The model under review builds one solid part; all positions refer to its coordinate system, in mm. A direction names the side the tool comes from. Coordinates: 2 decimals unless noted, no trailing zeros. Loops run counter-clockwise (first coordinate to the right, second up) from the corner with the lowest first, then second, coordinate; pieces in that order, holes last. Notation, with made-up numbers: (53, 71.5) - (92, 71.5) arc R15 cw to (92, 80.5) - close; hole circle Ø7 at (-7, 60.25). An arc over 180 degrees is marked (long way). One line per item, written item: value. Start each with the question number.
1. To check wall thickness, follow line 1 (X direction, y = 1.85, z = -15); line 2 (X direction, y = 2.3, z = -28); line 3 (Z direction, x = 22, y = 2.5). State the ranges of each line that lie inside material, in increasing order.
2. For faces 1 (the face through (10, 2, -2)), 2 (the face through (7.73, 2.03, -33.99)), 3 (the face through (4, 2, -23)), list the 3-axis set-ups (+Z, -Z, +X, -X, +Y, -Y) from which the entire face can be reached by the end or side of a thin tool; tool diameter is ignored.
3. Insertion check: P1, Ø2, axis at x = 22, y = 2.5, coming from the +Z side; P2, Ø1.2, axis at y = 2, z = -2, coming from the -X side; P3, Ø1.2, axis at y = 3, z = -6.5, coming from the +X side. Each pin has a flat end and moves straight along its axis. Give the tip position at first contact, or say it passes through.
4. We need section A-A, the plane z = -2. Give the boundary of the cut face in (x, y), then the cut area to 3 significant figures.
5. We need section B-B, the plane x = 15. Give the boundary of the cut face in (y, z).
6. Mouldability with a two-part tool opening along Z and no side actions: class faces 4 (the face through (29.14, 2.03, -42.1)), 5 (the face through (15, 2, 0)), 6 (the face through (15.07, 2.03, -29.5)), 7 (the face through (20, 2, -2)) as +Z half, -Z half, draft (parallel to the pull), parting line (faces both ways), or undercut.
7. We need section C-C, the plane x = 21.25. Give the boundary of the cut face in (y, z).
8. We need section D-D, the plane y = 1.8. Count the separate pieces of the cut face and the enclosed holes in it, then the cut area to 3 significant figures.
from build123d import *

# Parameters (mm, degrees)
SKETCH1_W           = 10
SKETCH1_H           = 4
SKETCH1_W_2         = 4
SKETCH1_H_2         = 10
BOSS_EXTRUDE1_DEPTH = 4
SKETCH3_W           = 30
SKETCH3_H           = 4
BOSS_EXTRUDE2_DEPTH = 13
SKETCH4_R           = 2.2
CUT_EXTRUDE2_DEPTH  = 10
FILLET1_R           = 3
FILLET2_R           = 4
SKETCH6_R           = 1.5
CUT_EXTRUDE3_DEPTH  = 10


with BuildPart() as part:
    # Sketch1 → Boss-Extrude1 (new body)
    with BuildSketch(Plane(origin=(0, 0, 0), x_dir=(1, 0, 0), z_dir=(0, 1, 0))):
        Polygon((4, 10), (4, 4), (10, 4), (20, 4), (26, 4), (26, 10), (26, 20), (26, 26), (20, 26), (10, 26), (4, 26), (4, 20), align=None)
        with Locations((15, 2)):
            Rectangle(SKETCH1_W, SKETCH1_H)
        with Locations((28, 15)):
            Rectangle(SKETCH1_W_2, SKETCH1_H_2)
        with Locations((15, 28)):
            Rectangle(SKETCH1_W, SKETCH1_H)
        with Locations((2, 15)):
            Rectangle(SKETCH1_W_2, SKETCH1_H_2)
    extrude(amount=BOSS_EXTRUDE1_DEPTH)

    # Sketch3 → Boss-Extrude2 (add)
    with BuildSketch(Plane(origin=(0, 0, -30), x_dir=(-1, 0, 0), z_dir=(0, 0, -1))):
        with Locations((-15, 2)):
            Rectangle(SKETCH3_W, SKETCH3_H)
    extrude(amount=BOSS_EXTRUDE2_DEPTH)

    # Sketch4 → Cut-Extrude2 (cut)
    with BuildSketch(Plane(origin=(0, 4, 0), x_dir=(1, 0, 0), z_dir=(0, 1, 0))):
        with Locations((24, 36.5)):
            Circle(SKETCH4_R)
        with Locations((6, 36.5)):
            Circle(SKETCH4_R)
        Polygon((9.146625176, 38.868807717), (3.631192283, 33.353374824), (2.853374824, 34.131192283), (8.368807717, 39.646625176), align=None)
        Polygon((21.684225292, 39.699658185), (27.199658185, 34.184225292), (26.315774708, 33.300341815), (20.800341815, 38.815774708), align=None)
        Polygon((8.368807717, 33.353374824), (9.146625176, 34.131192283), (3.631192283, 39.646625176), (2.853374824, 38.868807717), align=None)
        Polygon((20.800341815, 34.184225292), (21.684225292, 33.300341815), (27.199658185, 38.815774708), (26.315774708, 39.699658185), align=None)
    extrude(amount=-CUT_EXTRUDE2_DEPTH, mode=Mode.SUBTRACT)

    # Fillet1
    fillet1_edges = [part.edges().sort_by_distance(p)[0] for p in [
        (30, 2, -43),
        (0, 2, -43),
    ]]
    fillet(fillet1_edges, radius=FILLET1_R)

    # Fillet2
    fillet2_edges = [part.edges().sort_by_distance(p)[0] for p in [
        (30, 2, -30),
        (0, 2, -30),
    ]]
    fillet(fillet2_edges, radius=FILLET2_R)

    # Sketch6 → Cut-Extrude3 (cut)
    with BuildSketch(Plane(origin=(0, 4, 0), x_dir=(1, 0, 0), z_dir=(0, 1, 0))):
        with Locations(Location((28, 15, 0), (0, 0, 270))):
            Circle(SKETCH6_R)
        with Locations(Location((15, 2, 0), (0, 0, 270))):
            Circle(SKETCH6_R)
        with Locations(Location((2, 15, 0), (0, 0, 270))):
            Circle(SKETCH6_R)
        with Locations(Location((15, 28, 0), (0, 0, 270))):
            Circle(SKETCH6_R)
    extrude(amount=-CUT_EXTRUDE3_DEPTH, mode=Mode.SUBTRACT)


solid = part.part
Findings below:
1. line 1: 0 to 0.5, 3.5 to 26.5, 29.5 to 30
1. line 2: 10 to 13.5, 16.5 to 20
1. line 3: -43 to -39.38, -37.62 to -37.42, -35.58 to -35.38, -33.62 to -30, -26 to -4
2. face 1: +Z, -X, +Y, -Y
2. face 2: +Y, -Y
2. face 3: -X, +Y, -Y
3. P1: z = -4
3. P2: x = 10
3. P3: x = 26
4. outline: (10, 0) - (13.5, 0) - (13.5, 4) - (10, 4) - close; (16.5, 0) - (20, 0) - (20, 4) - (16.5, 4) - close
4. area: 28.0 mm2
5. outline: (0, -43) - (4, -43) - (4, -29.5) - (0, -29.5) - close; (0, -26.5) - (4, -26.5) - (4, -3.5) - (0, -3.5) - close; (0, -0.5) - (4, -0.5) - (4, 0) - (0, 0) - close
6. face 4: -Z half
6. face 5: +Z half
6. face 6: undercut
6. face 7: draft
7. outline: (0, -43) - (4, -43) - (4, -39.27) - (0, -39.27) - close; (0, -38.37) - (4, -38.37) - (4, -34.63) - (0, -34.63) - close; (0, -33.73) - (4, -33.73) - (4, -30) - (0, -30) - close; (0, -26) - (4, -26) - (4, -4) - (0, -4) - close
8. separate pieces: 1
8. enclosed holes: 6
8. area: 948 mm2
